The figure shows three views and two pictorial views of one solid part (mm, origin at its lowest corner). Answer the questions. A direction names the side the tool comes from. Give positions to 0.01 mm unless a question says otherwise; leave off trailing zeros. Write each loop counter-clockwise with the first axis right and the second up, starting at its lowest first coordinate (ties: lowest second). Pieces come first, ordered by that corner, then holes. Notation, with made-up numbers: (4, 73) - (28, 73) arc R21 cw to (28, 95) - close; hole circle Ø2 at (-22.75, 39.5). An arc over 180 degrees is marked (long way). Answer as CSV lines item,"result". Start each with the question number.
(1) Find section D-D (x = 46.5). Write down the section's boundary in (y, z), then the cut area to 3 significant figures.
(2) Each of these flat-tipped pins is pushed along its axis until it touches: pin 1 Ø6 at (y, z) = (30.5, 9.5) entering from -X; pin 2 Ø1 at (y, z) = (24.5, 9) entering from +X; pin 3 Ø1.5 at (x, y) = (61, 32) entering from +Z. Where does it stop, or does it pass through?
(3) For the marked faces 1 and 2, determine the directions among +Z, -Z, +X, -X, +Y, -Y from which every point of the face is accessible in a straight line to the end or side of a thin tool.
(4) Find section C-C (z = 10). Write down the section's boundary in (x, y) (1 decimal).
(5) Find section A-A (x = 71.5). Write down the section's boundary in (y, z).
(6) Straight lines are drawn through the part: probe 1 along Z at (x, y) = (53, 28); probe 2 along Y at (x, z) = (47, 6.25). For each, find the intervals that lie inside material, in ascending order.
(7) Find section B-B (y = 36). Write down the section's boundary in (x, z), then the cut area to 3 significant figures.
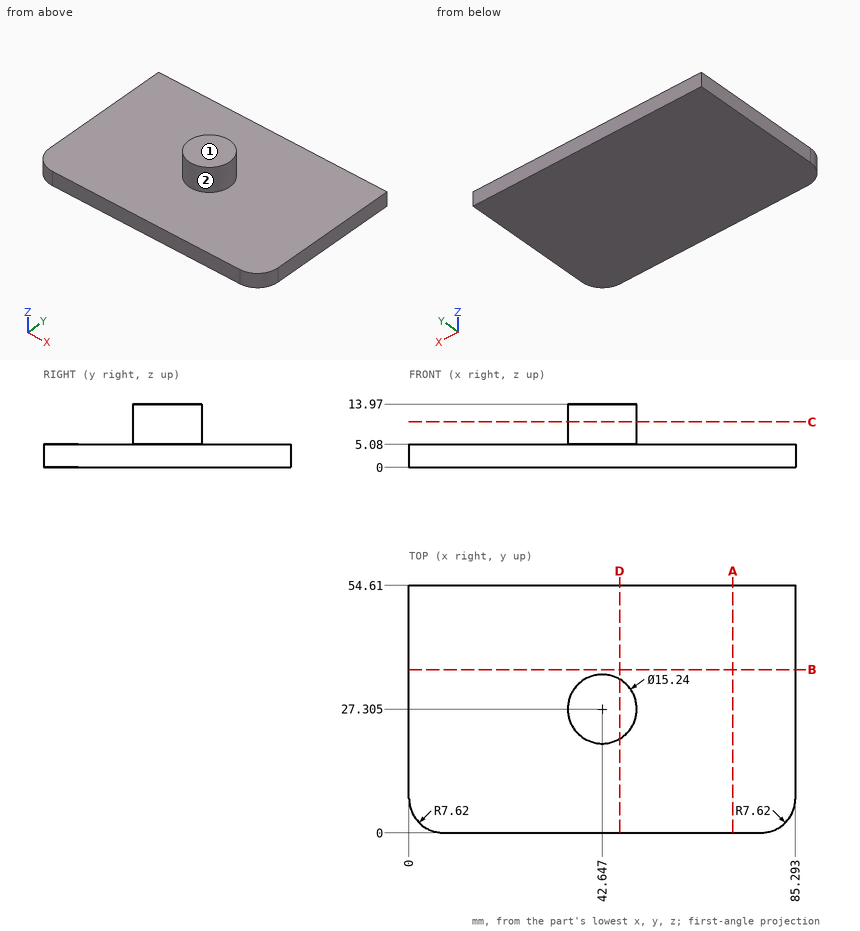
Result set:
1,outline,"(0, 0) - (54.61, 0) - (54.61, 5.08) - (33.88, 5.08) - (33.88, 13.97) - (20.73, 13.97) - (20.73, 5.08) - (0, 5.08) - close"
1,area,"394 mm^2"
2,pin 1,"x = 35.03"
2,pin 2,"x = 49.91"
2,pin 3,"z = 5.08"
3,face 1,"+Z, +X, -X, +Y, -Y"
3,face 2,"+Z"
4,outline,"circle Ø15.2 at (42.6, 27.3)"
5,outline,"(0, 0) - (54.61, 0) - (54.61, 5.08) - (0, 5.08) - close"
6,probe 1,"0 to 5.08"
6,probe 2,"21.05 to 33.56"
7,outline,"(0, 0) - (85.29, 0) - (85.29, 5.08) - (0, 5.08) - close"
7,area,"433 mm^2"
